Source: CAD feature listing. Evaluate the final solid. Frame: model axes, mm. Round coordinates to 2 decimals unless told otherwise and drop trailing zeros. Order: outer loops, then holes, each group sorted by start corner. A loop starts at its lowest first (then second) coordinate and runs counter-clockwise, first axis right, second up. Notation, with made-up numbers: (26, 80.5) -> (83, 80.5) arc R13 cw to (83, 86.5) -> close; hole circle Ø5 at (85.25, -10). An arc over 180 degrees is marked (long way). One line per item, written item: value. Start each with the question number.
1) Section B-B (z = -124). Return the cut outline in (x, y).
2) Section A-A (y = 2.5). State how many separate pieces and enclosed holes the cut face has, and give its area (3 significant figures).
3) Pin query (flat end, axial travel): P1, Ø0.9, axis at x = 250, y = 1.5, coming from the +Z side. Return the tip coordinate at first contact, or that it passes through.
4) Ray query, L1, parallel to X at y = 2.3, z = 60; L2, parallel to Z at x = -69.5, y = 1.55; L3, parallel to X at y = 0.25, z = 37. Return the intervals inside material, ascending.
5) Section C-C (z = -7). Return the cut outline in (x, y).
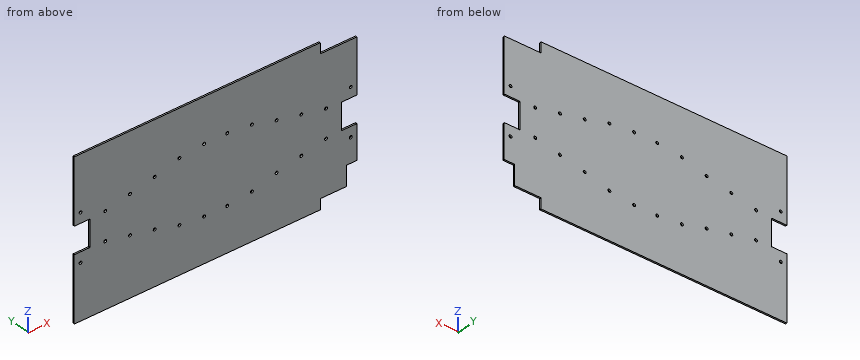
```python
from build123d import *

# Parameters (mm, degrees)
SKETCH1_W                  = 539
SKETCH1_H                  = 299
BOSS_EXTRUDE1_DEPTH        = 3
SKETCH5_W                  = 70
SKETCH5_H                  = 20
CUT_EXTRUDE2_DEPTH         = 309.203666429
SKETCH2_W                  = 30
SKETCH2_H                  = 51
CUT_EXTRUDE1_DEPTH         = 309.203666429
F_5_5_5_5_DIAMETER_HOLE1_D = 5.5
MIRROR3_COPY_1_D           = 5.5
FILLET1_R                  = 0.5


with BuildPart() as part:
    # Sketch1 → Boss-Extrude1 (new body)
    with BuildSketch(Plane(origin=(0, 0, 0), x_dir=(1, 0, 0), z_dir=(0, 1, 0))):
        Rectangle(SKETCH1_W, SKETCH1_H)
    extrude(amount=BOSS_EXTRUDE1_DEPTH)

    # Sketch5 → Cut-Extrude2 (cut, through all)
    with BuildSketch(Plane(origin=(0, 3, 0), x_dir=(1, 0, 0), z_dir=(0, 1, 0))):
        Polygon((269.5, 149.5), (199.5, 149.5), (199.5, 129.5), (249.5, 129.5), (249.5, 91.5), (269.5, 91.5), align=None)
        with Locations((234.5, -139.5)):
            Rectangle(SKETCH5_W, SKETCH5_H)
    extrude(amount=-CUT_EXTRUDE2_DEPTH, mode=Mode.SUBTRACT)

    # Sketch2 → Cut-Extrude1 (cut, through all)
    with BuildSketch(Plane(origin=(0, 3, 0), x_dir=(1, 0, 0), z_dir=(0, 1, 0))):
        with Locations((-254.5, 0)):
            Rectangle(SKETCH2_W, SKETCH2_H)
    cut_extrude1 = extrude(amount=-CUT_EXTRUDE1_DEPTH, mode=Mode.SUBTRACT)

    # Mirror1: Cut-Extrude1 across plane
    add(cut_extrude1.mirror(Plane(origin=(0, 0, 0), x_dir=(0, 0, 1), z_dir=(1, 0, 0))), mode=Mode.SUBTRACT)

    # Ø5.5 (5.5) Diameter Hole1 (through all)
    with Locations(Plane(origin=(-257.5, 3, 45), x_dir=(0, 0, 1), z_dir=(0, 1, 0))):
        with Locations((0, 0), (-18.019432511, 47.1), (-8.008018456, 94.2), (2.003395598, 141.3), (15, 188.4), (20, 235.5)):
            f_5_5_5_5_diameter_hole1 = Hole(F_5_5_5_5_DIAMETER_HOLE1_D / 2)

    # Mirror2: Ø5.5 (5.5) Diameter Hole1 across plane
    add(f_5_5_5_5_diameter_hole1.mirror(Plane(origin=(0, 0, 0), x_dir=(0, 0, 1), z_dir=(1, 0, 0))), mode=Mode.SUBTRACT)

    # Mirror3: Ø5.5 (5.5) Diameter Hole1 across plane
    add(f_5_5_5_5_diameter_hole1.mirror(Plane.XY), mode=Mode.SUBTRACT)

    # Mirror3 copy 1 (through all)
    with Locations(Plane(origin=(257.5, 3, -45), x_dir=(0, 0, -1), z_dir=(0, 1, 0))):
        with Locations((0, 0), (-18.019432511, 47.1), (-8.008018456, 94.2), (2.003395598, 141.3), (15, 188.4), (20, 235.5)):
            Hole(MIRROR3_COPY_1_D / 2)

    # Fillet1
    fillet1_edges = [part.edges().sort_by_distance(p)[0] for p in [
        (269.5, 1.5, -91.5),
        (249.5, 1.5, -91.5),
        (249.5, 1.5, -129.5),
        (199.5, 1.5, -129.5),
        (199.5, 1.5, -149.5),
        (269.5, 1.5, 129.5),
        (199.5, 1.5, 149.5),
        (199.5, 1.5, 129.5),
        (-269.5, 1.5, 25.5),
        (-269.5, 1.5, -25.5),
        (-239.5, 1.5, -25.5),
        (-239.5, 1.5, 25.5),
        (269.5, 1.5, -25.5),
        (269.5, 1.5, 25.5),
        (239.5, 1.5, 25.5),
        (239.5, 1.5, -25.5),
        (-269.5, 1.5, -149.5),
        (-269.5, 1.5, 149.5),
    ]]
    fillet(fillet1_edges, radius=FILLET1_R)


solid = part.part
```
Findings:
1. outline: (-269.5, 0) -> (249.5, 0) -> (249.5, 3) -> (-269.5, 3) -> close
2. separate pieces: 1
2. enclosed holes: 24
2. area: 154,000 mm2
3. P1: z = 129.5
4. L1: -269.5 to -71.85, -66.35 to 66.35, 71.85 to 269.5
4. L2: -149.5 to -62.72, -57.28 to 57.28, 62.72 to 149.5
4. L3: -269.5 to -166.05, -160.55 to 160.55, 166.05 to 269.5
5. outline: (-239.5, 0) -> (239.5, 0) -> (239.5, 3) -> (-239.5, 3) -> close
